Model file for the job. Use its own axes, mm. Face numbers are marked on the shaded views. A direction names the side the tool comes from. Round coordinates to 2 decimals unless told otherwise and drop trailing zeros. Loops run counter-clockwise (first coordinate to the right, second up) from the corner with the lowest first, then second, coordinate; pieces in that order, holes last. Notation, with made-up numbers: (58, 8.25) -> (108, 8.25) arc R16 ccw to (108, 23.25) -> close; hole circle Ø11 at (46.25, 37). An arc over 180 degrees is marked (long way). Use a Markdown table: item, result.
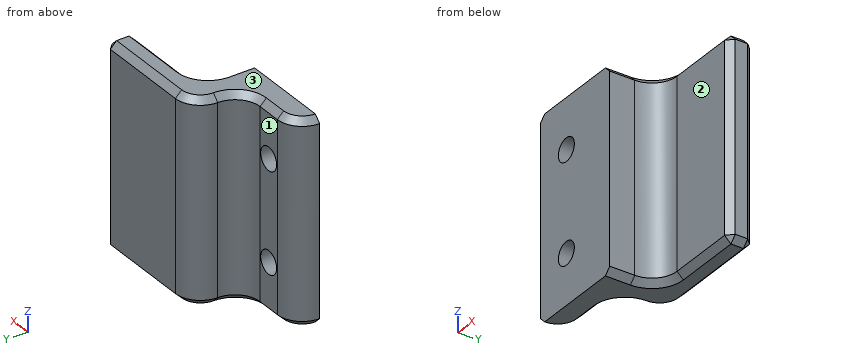
from build123d import *

# Parameters (mm, degrees)
BOSS_EXTRUDE1_DEPTH = 25.5
SKETCH3_R           = 2.921
CUT_EXTRUDE1_DEPTH  = 41.331656301
FILLET1_START       = -25.5
FILLET1_DEPTH       = 51
FILLET1_2_DEPTH     = 51
CHAMFER1_SIZE       = 1.5875


with BuildPart() as part:
    # Sketch1 → Boss-Extrude1 (new, symmetric)
    with BuildSketch(Plane.XY):
        Polygon((-22.2, -9.525), (3.2, -9.525), (3.2, 3.175), (28.55, 3.175), (28.55, 9.525), (-3.2, 9.525), (-3.2, -3.175), (-22.2, -3.175), align=None)
    extrude(amount=BOSS_EXTRUDE1_DEPTH, both=True)

    # Sketch3 → Cut-Extrude1 (cut, through all)
    with BuildSketch(Plane(origin=(0, -3.175, 0), x_dir=(1, 0, 0), z_dir=(0, 1, 0))):
        with Locations(Location((-12.675, -12.7, 0), (0, 0, 180))):
            Circle(SKETCH3_R)
    cut_extrude1 = extrude(amount=-CUT_EXTRUDE1_DEPTH, mode=Mode.SUBTRACT)

    # Mirror1: Cut-Extrude1 across plane
    add(cut_extrude1.mirror(Plane.XY), mode=Mode.SUBTRACT)

    # Fillet1: read off the stored shape, not the designer's step
    # Fillet1 outline → Fillet1 (cut)
    with BuildSketch(Plane.XY.offset(FILLET1_START)):
        with BuildLine():
            Line((-22.2, -3.175), (-22.2, -9.525))
            ThreePointArc((-22.2, -9.525), (-20.340128061, -5.034871939), (-15.85, -3.175))
            Line((-15.85, -3.175), (-22.2, -3.175))
        make_face()
        with BuildLine():
            Line((-3.2, 9.525), (-3.2, 3.175))
            ThreePointArc((-3.2, 3.175), (-1.340128061, 7.665128061), (3.15, 9.525))
            Line((3.15, 9.525), (-3.2, 9.525))
        make_face()
    extrude(amount=FILLET1_DEPTH, mode=Mode.SUBTRACT)

    # Fillet1 2 outline → Fillet1 2 (add)
    with BuildSketch(Plane.XY.offset(FILLET1_START)):
        with BuildLine():
            ThreePointArc((3.2, -3.175), (5.059871939, 1.315128061), (9.55, 3.175))
            Line((9.55, 3.175), (3.2, 3.175))
            Line((3.2, 3.175), (3.2, -3.175))
        make_face()
        with BuildLine():
            ThreePointArc((-3.2, 3.175), (-5.059871939, -1.315128061), (-9.55, -3.175))
            Line((-9.55, -3.175), (-3.2, -3.175))
            Line((-3.2, -3.175), (-3.2, 3.175))
        make_face()
    extrude(amount=FILLET1_2_DEPTH)

    # Chamfer1
    chamfer1_edges = [part.edges().sort_by_distance(p)[0] for p in [
        (3.2, -6.35, -25.5),
        (3.2, -6.35, 25.5),
        (28.55, 9.525, 0),
        (28.55, 3.175, 0),
        (28.55, 6.35, 25.5),
        (15.85, 9.525, 25.5),
        (19.05, 3.175, -25.5),
        (19.05, 3.175, 25.5),
        (-12.7, -3.175, -25.5),
        (-1.340128061, 7.665128061, -25.5),
        (-20.340128061, -5.034871939, -25.5),
        (-12.7, -3.175, 25.5),
        (-1.340128061, 7.665128061, 25.5),
        (-20.340128061, -5.034871939, 25.5),
        (5.059871939, 1.315128061, -25.5),
        (5.059871939, 1.315128061, 25.5),
        (-5.059871939, -1.315128061, -25.5),
        (-5.059871939, -1.315128061, 25.5),
        (15.85, 9.525, -25.5),
        (28.55, 6.35, -25.5),
    ]]
    chamfer(chamfer1_edges, length=CHAMFER1_SIZE)


solid = part.part
Q1. Band-saw the part on C-C, the plane y = -6.25. Give the number of separate pieces and of enclosed holes in the cut face, plus the area to 3 significant figures.
Results list:
| item | result |
|---|---|
| separate pieces | 1 |
| enclosed holes | 2 |
| area | 1,190 mm² |
Q2. Band-saw the part on B-B, the plane x = 17. Give the cut face in (y, z) (1 decimal), plus the area to 3 significant figures.
Results list:
| item | result |
|---|---|
| outline | (3.2, -23.9) -> (4.8, -25.5) -> (7.9, -25.5) -> (9.5, -23.9) -> (9.5, 23.9) -> (7.9, 25.5) -> (4.8, 25.5) -> (3.2, 23.9) -> close |
| area | 319 mm² |
Q3. Drill centre lines: L1, parallel to X at y = -5, z = -12.7; L2, parallel to Y at x = -13, z = 6 (3 decimals); L3, parallel to X at y = -6, z = -12.7. Where is each one in solid material? Low to high. Write a range as from..to.
Results list:
| item | result |
|---|---|
| L1 | x = -20.3..-15.6, -9.75..3.2 |
| L2 | y = -9.525..-3.175 |
| L3 | x = -21.13..-15.6, -9.75..3.2 |
Q4. Flat gauge pins, fed straight in: pin 1 (1.5 mm diameter, centred on y = -4, z = -4.5, fed in from +X); pin 2 (8.5 mm diameter, centred on x = 19, z = 9.5, fed in from -Y) (3 decimals); pin 3 (7.5 mm diameter, centred on x = -12.675, z = 12.7, fed in from +Y). Where does each tip first touch, or does it go through?
Results list:
| item | result |
|---|---|
| pin 1 | stops at x = 3.2 |
| pin 2 | stops at y = 3.175 |
| pin 3 | stops at y = -3.14 |
Q5. Tool access for the marked faces 1, 2 and 3: list every direction of +Z, -Z, +X, -X, +Y, -Y with a clear straight run to the whole face (end or side of a thin tool).
Results list:
| item | result |
|---|---|
| face 1 | +Z, -Z, -X, +Y |
| face 2 | +Z, -Z, +X, -Y |
| face 3 | +Z, +X, -X, +Y, -Y |
